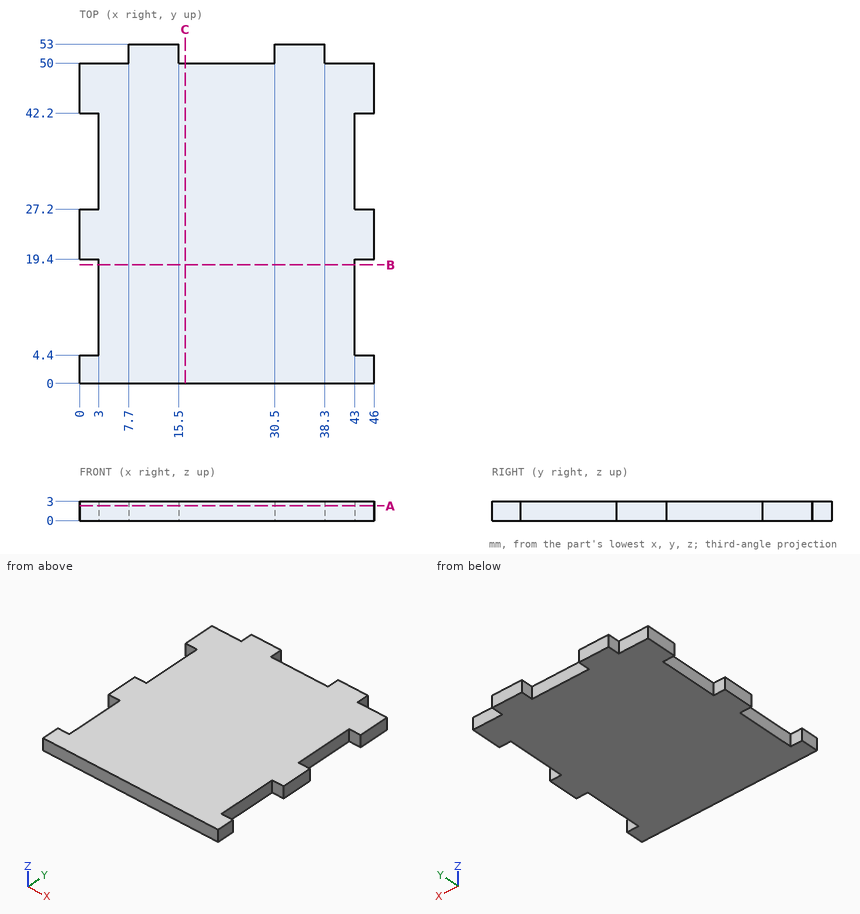
The drawing under review shows one solid part. Ordinate dimensions are in mm from its lowest x, y, z. Round coordinates to 2 decimals unless told otherwise and drop trailing zeros. Loops run counter-clockwise (first coordinate to the right, second up) from the corner with the lowest first, then second, coordinate; pieces in that order, holes last. Notation, with made-up numbers: (24, 58) -> (45, 58) arc R13 ccw to (45, 73) -> close; hole circle Ø3 at (-27.5, 21.25). An arc over 180 degrees is marked (long way). Answer in a Markdown table with one row per item.
1) Wall thickness on line 1 along Y through (x, z) = (44.5, 1.8); line 2 along X through (y, z) = (27.5, 2.5); line 3 along X through (y, z) = (51.5, 2.2): over which ranges is each line inside the solid? List them lowest first.
Taken from the geometry:
| item | result |
|---|---|
| line 1 | y = 0 to 4.4, 19.4 to 27.2, 42.2 to 50 |
| line 2 | x = 3 to 43 |
| line 3 | x = 7.7 to 15.5, 30.5 to 38.3 |
2) For pin 1 Ø0.9 at (x, z) = (44, 1.5) entering from +Y; pin 2 Ø1.5 at (y, z) = (52, 1.5) entering from -X; pin 3 Ø1.5 at (y, z) = (18.5, 2.5) entering from +X, all flat-tipped, find the tip position at first contact; note any pin that passes through.
Taken from the geometry:
| item | result |
|---|---|
| pin 1 | stops at y = 50 |
| pin 2 | stops at x = 7.7 |
| pin 3 | stops at x = 43 |
3) Consider section C-C, the plane x = 16.5. Write out the cut boundary in (y, z).
Taken from the geometry:
| item | result |
|---|---|
| outline | (0, 0) -> (50, 0) -> (50, 3) -> (0, 3) -> close |
4) Consider section B-B, the plane y = 18.5. Write out the cut boundary in (x, z).
Taken from the geometry:
| item | result |
|---|---|
| outline | (3, 0) -> (43, 0) -> (43, 3) -> (3, 3) -> close |
5) Consider section A-A, the plane z = 2.3. Write out the cut boundary in (x, y).
Taken from the geometry:
| item | result |
|---|---|
| outline | (0, 0) -> (46, 0) -> (46, 4.4) -> (43, 4.4) -> (43, 19.4) -> (46, 19.4) -> (46, 27.2) -> (43, 27.2) -> (43, 42.2) -> (46, 42.2) -> (46, 50) -> (38.3, 50) -> (38.3, 53) -> (30.5, 53) -> (30.5, 50) -> (15.5, 50) -> (15.5, 53) -> (7.7, 53) -> (7.7, 50) -> (0, 50) -> (0, 42.2) -> (3, 42.2) -> (3, 27.2) -> (0, 27.2) -> (0, 19.4) -> (3, 19.4) -> (3, 4.4) -> (0, 4.4) -> close |
